Model file for the job. Use its own axes, mm. A direction names the side the tool comes from. Coordinates: 2 decimals unless noted, no trailing zeros. Order: outer loops, then holes, each group sorted by start corner. A loop starts at its lowest first (then second) coordinate and runs counter-clockwise, first axis right, second up.
Autodesk Inventor part; units mm, degrees
ref_plane "YZ Plane" through (0, 0, 0) normal (1, 0, 0) x (0, 1, 0)
ref_plane "XZ Plane" through (0, 0, 0) normal (0, 1, 0) x (-1, 0, 0)
ref_plane "XY Plane" through (0, 0, 0) normal (0, 0, 1) x (1, 0, 0)
sketch "Sketch1" plane through (0, 0, 0) normal (0, 1, 0) x (-1, 0, 0)
  line L0 (0, 0) -> (155, 0)
  line L1 (155, 0) -> (155, -125)
  line L2 (155, -125) -> (0, -125)
  line L3 (0, -125) -> (0, 0)
  dimension "d0" = 125
  dimension "d1" = 155
extrude "Extrusion1" add sketch "Sketch1" along normal blind 60
sketch "Sketch2" plane through (0, 60, 0) normal (0, 1, 0) x (1, 0, 0)
  line L0 (-150, 5) -> (-5, 5)
  line L1 (-5, 5) -> (-5, 120)
  line L2 (-5, 120) -> (-150, 120)
  line L3 (-150, 120) -> (-150, 5)
  line L4 (-155, 0) -> (0, 0)
  line L5 (0, 125) -> (-155, 125)
  line L6 (-155, 125) -> (-155, 0)
  line L7 (0, 0) -> (0, 125)
  point P0 (-77.5, 125)
  dimension "d4" = 5
  dimension "d5" = 5
  dimension "d6" = 5
  dimension "d7" = 5
extrude "Extrusion2" cut sketch "Sketch2" against normal blind 55 contours L3 L2 L1 L0
sketch "Sketch3" plane through (0, 60, 0) normal (0, 1, 0) x (1, 0, 0)
  line L0 (-155, 0) -> (0, 0)
  line L1 (-155, 0) -> (0, 0)
  line L2 (0, 0) -> (0, 125)
  line L3 (0, 125) -> (-155, 125)
  line L4 (-155, 125) -> (-155, 0)
extrude "Extrusion3" add sketch "Sketch3" along normal blind 5
sketch "Sketch4" plane through (0, 65, 0) normal (0, 1, 0) x (1, 0, 0)
  circle A0 centre (-30, 95) radius 5
  line L0 (0, 125) -> (-155, 125)
  line L1 (0, 0) -> (0, 125)
  dimension "d12" = 10
  dimension "d13" = 30
  dimension "d14" = 30
extrude "Extrusion4" cut sketch "Sketch4" against normal blind 5
sketch "Sketch5" plane through (-155, 0, 0) normal (0, 0, 1) x (1, 0, 0)
  circle A0 centre (20, 20) radius 5
  line L0 (0, 0) -> (155, 0)
  line L1 (0, 0) -> (0, 65)
  dimension "d17" = 20
  dimension "d18" = 20
  dimension "d19" = 10
extrude "Extrusion5" cut sketch "Sketch5" against normal blind 20
sketch "Sketch6" plane through (0, 65, 0) normal (0, 1, 0) x (1, 0, 0)
  line L0 (-145, 5) -> (-105, 5)
  line L1 (-105, 5) -> (-105, 120)
  line L2 (-105, 120) -> (-145, 120)
  line L3 (-145, 120) -> (-145, 5)
  line L4 (-155, 125) -> (-155, 0)
  line L5 (0, 125) -> (-155, 125)
  line L6 (-155, 0) -> (0, 0)
  point P0 (-125, 5)
  dimension "d22" = 10
  dimension "d23" = 5
  dimension "d24" = 5
  dimension "d25" = 40
extrude "Extrusion6" cut sketch "Sketch6" against normal blind 5
sketch "Sketch7" plane through (-155, 0, 0) normal (0, 0, 1) x (1, 0, 0)
  circle A0 centre (20, 30) radius 1.5
  circle A1 centre (20, 20) radius 5
  circle A2 centre (20, 20) radius 5
  circle A3 centre (10, 20) radius 1.5
  circle A4 centre (20, 10) radius 1.5
  circle A5 centre (30, 20) radius 1.5
  point P0 (155, 0)
  dimension "d28" = 3
  dimension "d31" = 360
  dimension "d35" = 10
extrude "Extrusion7" cut sketch "Sketch7" against normal blind 5 contours A0 | A3 | A4 | A5
sketch "Sketch8" plane through (0, 65, 0) normal (0, 1, 0) x (1, 0, 0)
  point P0 (0, 0)
sketch "Sketch9" plane through (0, 65, 0) normal (0, 1, 0) x (1, 0, 0)
  point P0 (0, 0)
sketch "Sketch10" plane through (0, 65, 0) normal (0, 1, 0) x (1, 0, 0)
  point P0 (0, 0)
sketch "Sketch11" plane through (0, 65, 0) normal (0, 1, 0) x (1, 0, 0)
  circle A0 centre (-40, 95) radius 1.5
  circle A1 centre (-30, 95) radius 5
  circle A2 centre (-30, 95) radius 5
  circle A3 centre (-30, 85) radius 1.5
  circle A4 centre (-20, 95) radius 1.5
  circle A5 centre (-30, 105) radius 1.5
  point P0 (0, 0)
  dimension "d36" = 10
  dimension "d37" = 3
  dimension "d40" = 360
extrude "Extrusion8" cut sketch "Sketch11" against normal blind 5 contours A0 | A3 | A4 | A5
chamfer "Chamfer1" distance 1 angle 45 8 edges at (-31.5, 65, -105) (-21.5, 65, -95) (-31.5, 65, -85) (-41.5, 65, -95) (-126.5, 20, 0) (-136.5, 30, 0) (-136.5, 10, 0) (-146.5, 20, 0)
chamfer "Chamfer3" distance 1 angle 45 4 edges at (-105, 65, -62.5) (-125, 65, -120) (-145, 65, -62.5) (-125, 65, -5)
sketch "Sketch12" plane through (-5, 5, -5) normal (0, 0, -1) x (-1, 0, 0)
  line L0 (0, 0) -> (145, 0)
  line L1 (145, 0) -> (115, 0)
  line L2 (115, 0) -> (115, 30)
  line L3 (115, 30) -> (145, 30)
  line L4 (145, 30) -> (145, 0)
  point P0 (-5, -5)
  point P1 (115, 0)
  dimension "d53" = 30
  dimension "d54" = 30
extrude "Extrusion9" add sketch "Sketch12" along normal blind 5
sketch "Sketch13" plane through (-155, 0, 0) normal (0, 0, 1) x (1, 0, 0)
  point P0 (155, 0)
sketch "Sketch14" plane through (-135, 20, -5) normal (0, 0, 1) x (1, 0, 0)
  circle A0 centre (0, 0) radius 5
  point P0 (135, -20)
extrude "Extrusion10" cut sketch "Sketch14" against normal blind 20
chamfer "Chamfer4" distance 1 angle 45 2 edges at (-35, 65, -95) (-140, 20, 0)
chamfer "Chamfer5" distance 3 angle 45 12 edges at (0, 65, -62.5) (-77.5, 65, 0) (-155, 65, -62.5) (-77.5, 65, -125) (0, 32.5, 0) (0, 32.5, -125) (-155, 32.5, -125) (-155, 32.5, 0) (0, 0, -62.5) (-77.5, 0, -125) (-155, 0, -62.5) (-77.5, 0, 0)
sketch "Sketch15" plane through (0, 65, 0) normal (0, 1, 0) x (1, 0, 0)
  point P0 (0, 0)
sketch "Sketch16" plane through (0, 65, 0) normal (0, 1, 0) x (1, 0, 0)
  point P0 (0, 0)
properties part number "Water container"
Q1. Probe line 1 (Z direction, x = -30, y = 61.1); line 2 (Z direction, x = -64.5, y = 56.5); line 3 (X direction, y = 21, z = -60.5). List the from-to ranges inside material, lowest first.
Established:
line 1: z = -125 to -106.5, -103.5 to -100, -90 to -86.5, -83.5 to 0
line 2: z = -125 to -120, -5 to 0
line 3: x = -155 to -150, -5 to 0
Q2. Cut at C-C, the plane z = -69.5. List the corners of the cut face in (x, y), plus the area to 3 significant figures.
Established:
outline: (-155, 3) - (-152, 0) - (-3, 0) - (0, 3) - (0, 62) - (-3, 65) - (-104, 65) - (-105, 64) - (-105, 60) - (-5, 60) - (-5, 5) - (-150, 5) - (-150, 60) - (-145, 60) - (-145, 64) - (-146, 65) - (-152, 65) - (-155, 62) - close
area: 1,880 mm2
Q3. Cut at A-A, the plane x = -64.5. List the corners of the cut face in (y, z).
Established:
outline: (0, -122) - (3, -125) - (62, -125) - (65, -122) - (65, -3) - (62, 0) - (3, 0) - (0, -3) - close; hole (5, -120) - (60, -120) - (60, -5) - (5, -5) - close
Q4. Cut at B-B, the plane y = 57. List the corners of the cut face in (x, z), plus the area to 3 significant figures.
Established:
outline: (-155, -122) - (-152, -125) - (-3, -125) - (0, -122) - (0, -3) - (-3, 0) - (-152, 0) - (-155, -3) - close; hole (-150, -120) - (-5, -120) - (-5, -5) - (-150, -5) - close
area: 2,680 mm2
Q5. Drop flat-ended pins along their axis: P1, Ø6, axis at x = -125.5, z = -68, coming from the +Y side; P2, Ø1.5, axis at x = -134.5, y = 9.5, coming from the +Z side. Give the stop position or say it passes through.
Established:
P1: stops at y = 5
P2: stops at z = -5
Q6. Mould opens along Z. For faces 1 (the face through (-62, 65, -63)), 2 (the face through (-5, 33, -62)), 3 (the face through (-79, 32, 0)) say: pulls with the +Z half, pulls with the -Z half, needs draft (parallel to the pull), parting line crosses it, or undercut.
Established:
face 1: needs draft
face 2: undercut
face 3: pulls with the +Z half
Q7. Which spindle directions (+Z, -Z, +X, -X, +Y, -Y) get a long thin tool onto all of the face, cutting with end or side? Do faces 4 (the face through (-155, 32, -63)), 5 (the face through (-79, 35, -5)), 6 (the face through (-31.08, 62.03, -90.12)). Say none if no direction does.
Established:
face 4: +Z, -Z, -X, +Y, -Y
face 5: none
face 6: +Y
